from build123d import *

# Parameters (mm, degrees)
CROQUIS1_W                                           = 108
CROQUIS1_H                                           = 100
SALIENTE_EXTRUIR2_DEPTH                              = 2
CROQUIS3_W                                           = 108
CROQUIS3_H                                           = 2
SALIENTE_EXTRUIR3_DEPTH                              = 90
CORTAR_EXTRUIR1_DEPTH                                = 90
TALADRO_DE_MARGEN_PARA_M42_D                         = 4.5
TALADRO_DE_MARGEN_PARA_M42_DEPTH                     = 10
TALADRO_DE_MARGEN_PARA_M42_TIP                       = 1.351936393
SALIENTE_EXTRUIR4_DEPTH                              = 2
SALIENTE_EXTRUIR5_DEPTH                              = 2
REFRENTADO_PARA_TORNILLO_CON_CABEZA_TRON_D           = 1.778
REFRENTADO_PARA_TORNILLO_CON_CABEZA_TRON_DEPTH       = 10
REFRENTADO_PARA_TORNILLO_CON_CABEZA_TRON_CBORE_D     = 3.57124
REFRENTADO_PARA_TORNILLO_CON_CABEZA_TRON_CBORE_DEPTH = 1.1176
REFRENTADO_PARA_TORNILLO_CON_CABEZA_TRON_TIP         = 0.53416509


with BuildPart() as part:
    # Croquis1 → Saliente-Extruir2 (new body)
    with BuildSketch(Plane(origin=(0, 0, 0), x_dir=(1, 0, 0), z_dir=(0, 1, 0))):
        Rectangle(CROQUIS1_W, CROQUIS1_H)
    extrude(amount=SALIENTE_EXTRUIR2_DEPTH)

    # Croquis3 → Saliente-Extruir3 (add)
    with BuildSketch(Plane(origin=(0, 2, 0), x_dir=(1, 0, 0), z_dir=(0, 1, 0))):
        with Locations((0, 49)):
            Rectangle(CROQUIS3_W, CROQUIS3_H)
    extrude(amount=SALIENTE_EXTRUIR3_DEPTH)

    # Croquis4 → Cortar-Extruir1 (cut)
    with BuildSketch(Plane.XY.offset(-48)):
        with BuildLine():
            Line((-7, 92), (7, 92))
            ThreePointArc((7, 92), (0, 85), (-7, 92))
        make_face()
    extrude(amount=-CORTAR_EXTRUIR1_DEPTH, mode=Mode.SUBTRACT)

    # Taladro de margen para M42
    with Locations(Plane(origin=(0, 0, 0), x_dir=(-1, 0, 0), z_dir=(0, -1, 0))):
        with Locations((0, 20), (-20, 0), (0, -20), (20, 0), (0, 0)):
            Hole(TALADRO_DE_MARGEN_PARA_M42_D / 2, depth=TALADRO_DE_MARGEN_PARA_M42_DEPTH)
            with Locations((0, 0, -(TALADRO_DE_MARGEN_PARA_M42_DEPTH + TALADRO_DE_MARGEN_PARA_M42_TIP / 2))):  # 118° drill point
                Cone(0, TALADRO_DE_MARGEN_PARA_M42_D / 2, TALADRO_DE_MARGEN_PARA_M42_TIP, mode=Mode.SUBTRACT)

    # Croquis19 → Saliente-Extruir4 (add)
    with BuildSketch(Plane(origin=(54, 0, 0), x_dir=(0, 0, -1), z_dir=(1, 0, 0))):
        Polygon((48, 92), (-50, 2), (48, 2), align=None)
    extrude(amount=-SALIENTE_EXTRUIR4_DEPTH)

    # Croquis20 → Saliente-Extruir5 (add)
    with BuildSketch(Plane.ZY.offset(54)):
        Polygon((50, 2), (-48, 2), (-48, 92), align=None)
    extrude(amount=-SALIENTE_EXTRUIR5_DEPTH)

    # Refrentado para tornillo con cabeza troncocónica de #01
    with Locations(Plane.XY.offset(-48)):
        with Locations((-23.335241647, 67.193959118), (23.34076456, 67.198738562), (-23.269344277, 26.863067453), (23.181350949, 26.939215525)):
            CounterBoreHole(REFRENTADO_PARA_TORNILLO_CON_CABEZA_TRON_D / 2, REFRENTADO_PARA_TORNILLO_CON_CABEZA_TRON_CBORE_D / 2, REFRENTADO_PARA_TORNILLO_CON_CABEZA_TRON_CBORE_DEPTH, depth=REFRENTADO_PARA_TORNILLO_CON_CABEZA_TRON_DEPTH)
            with Locations((0, 0, -(REFRENTADO_PARA_TORNILLO_CON_CABEZA_TRON_DEPTH + REFRENTADO_PARA_TORNILLO_CON_CABEZA_TRON_TIP / 2))):  # 118° drill point
                Cone(0, REFRENTADO_PARA_TORNILLO_CON_CABEZA_TRON_D / 2, REFRENTADO_PARA_TORNILLO_CON_CABEZA_TRON_TIP, mode=Mode.SUBTRACT)


solid = part.part
Source: CAD feature listing. Evaluate the final solid. Frame: model axes, mm. A direction names the side the tool comes from. Round coordinates to 2 decimals unless told otherwise and drop trailing zeros. Order: outer loops, then holes, each group sorted by start corner. A loop starts at its lowest first (then second) coordinate and runs counter-clockwise, first axis right, second up. Notation, with made-up numbers: (78.5, 59) -> (125.5, 59) arc R31 ccw to (125.5, 87) -> close; hole circle Ø8 at (28, 78.5). An arc over 180 degrees is marked (long way). Answer as CSV lines item,"result".
Item 1: Section C-C, the plane z = 0. Return loops of the section in (x, y), plus the area to 3 significant figures.
A:
outline,"(-54, 0) -> (-22.25, 0) -> (-22.25, 2) -> (-52, 2) -> (-52, 47.92) -> (-54, 47.92) -> close; (-17.75, 0) -> (-2.25, 0) -> (-2.25, 2) -> (-17.75, 2) -> close; (2.25, 0) -> (17.75, 0) -> (17.75, 2) -> (2.25, 2) -> close; (22.25, 0) -> (54, 0) -> (54, 47.92) -> (52, 47.92) -> (52, 2) -> (22.25, 2) -> close"
area,"373 mm²"
Item 2: Pin query (flat end, axial travel): pin 1 Ø3 at (x, y) = (-23.34, 67.19) entering from +Z; pin 2 Ø12 at (x, z) = (14.5, 5.5) entering from +Y; pin 3 Ø6 at (x, y) = (-31.5, 23) entering from +Z. Return the tip coordinate at first contact, or that it passes through.
A:
pin 1,"z = -49.12"
pin 2,"y = 2"
pin 3,"z = -48"
Item 3: Reachability of faces 4 (the face through (54, 36, -10)), 5 (the face through (-23.72, 65.45, -48.55)), 6 (the face through (52, 28, -20)) from +Z, -Z, +X, -X, +Y, -Y: full face, straight path, thin tool, end or side. Return the list, or none.
A:
face 4,"+Z, -Z, +X, +Y, -Y"
face 5,"+Z"
face 6,"+Z, +Y"
Item 4: Line query: L1, parallel to Z at x = 0, y = 1.5; L2, parallel to X at y = 26.5, z = -43.5; L3, parallel to Y at x = 34, z = 5.5. Output: solid intervals per line, ascending.
A:
L1,"-50 to -22.25, -17.75 to -2.25, 2.25 to 17.75, 22.25 to 50"
L2,"-54 to -52, 52 to 54"
L3,"0 to 2"
Item 5: Section D-D, the plane x = 0. Return loops of the section in (y, z), plus the area to 3 significant figures.
A:
outline,"(0, -50) -> (85, -50) -> (85, -48) -> (2, -48) -> (2, -22.25) -> (0, -22.25) -> close; (0, -17.75) -> (2, -17.75) -> (2, -2.25) -> (0, -2.25) -> close; (0, 2.25) -> (2, 2.25) -> (2, 17.75) -> (0, 17.75) -> close; (0, 22.25) -> (2, 22.25) -> (2, 50) -> (0, 50) -> close"
area,"339 mm²"
Item 6: Section B-B, the plane z = 20. Return loops of the section in (x, y), plus the area to 3 significant figures.
A:
outline,"(-54, 0) -> (-2.25, 0) -> (-2.25, 2) -> (-52, 2) -> (-52, 29.55) -> (-54, 29.55) -> close; (2.25, 0) -> (54, 0) -> (54, 29.55) -> (52, 29.55) -> (52, 2) -> (2.25, 2) -> close"
area,"317 mm²"
Item 7: Pull-direction query (Z, two-part tool) for faces 1 (the face through (22.146, 1.014, -0.676)), 2 (the face through (22, 27, -49.118)), 3 (the face through (0, 85, -49)); classes: pulls with the +Z half, pulls with the -Z half, needs draft (parallel to the pull), parting line crosses it, or undercut.
A:
face 1,"undercut"
face 2,"pulls with the +Z half"
face 3,"needs draft"
Item 8: Section A-A, the plane x = -20. Return loops of the section in (y, z).
A:
outline,"(0, -50) -> (92, -50) -> (92, -48) -> (2, -48) -> (2, -2.25) -> (0, -2.25) -> close; (0, 2.25) -> (2, 2.25) -> (2, 50) -> (0, 50) -> close"
